from build123d import *

# Parameters (mm, degrees)
F1_DEPTH    = 2.5
F3_DEPTH    = 2.7
F4_R        = 1
F5_R        = 5
F7_R        = 2
F8_DEPTH    = 1
F6_W        = 8
F6_H        = 15
F9_DEPTH    = 1.1
F10_SIZE2   = 1.09999
F10_SIZE    = 14.99999
F10_2_SIZE2 = 1.09999
F10_2_SIZE  = 14.99999
F13_W       = 4
F13_H       = 4
F14_DEPTH   = 2


# Not quite as in the source:
# - a fillet or chamfer that OpenCascade refuses, or shapes differently, is made with other operations: its cross-section is extruded or revolved along the edge and cut away or added
# - two fillets or chamfers of one size are made in one step
# - a fillet or chamfer is up to 0.001 mm smaller than in the source, because OpenCascade refuses the exact size


with BuildPart() as f1:
    # F0 (on Top) → F1 (new body)
    with BuildSketch(Plane.XY):
        Polygon((55, 0), (4, 0), (0, -10), (0, -47), (59, -47), (59, -10), align=None)
    extrude(amount=F1_DEPTH)

    # F2 (on face) → F3 (join)
    with BuildSketch(Plane.XY.offset(2.5)):
        with BuildLine():
            Line((0, -39.5), (0, -47))
            Line((0, -47), (59, -47))
            Line((59, -47), (59, -39.5))
            Line((59, -39.5), (53.5, -32))
            Line((53.5, -32), (53.5, -4))
            ThreePointArc((53.5, -4), (52.3284271247, -1.1715728753), (49.5, 0))
            Line((49.5, 0), (9.5, 0))
            ThreePointArc((9.5, 0), (6.6715728753, -1.1715728753), (5.5, -4))
            Line((5.5, -4), (5.5, -32))
            Line((5.5, -32), (0, -39.5))
        make_face()
    extrude(amount=F3_DEPTH)

    # F4
    f4_edges = [f1.edges().sort_by_distance(p)[0] for p in [
        (0, -47, 2.6),
        (59, -47, 2.6),
        (4, 0, 1.25),
        (55, 0, 1.25),
        (59, -10, 1.25),
        (0, -10, 1.25),
    ]]
    fillet(f4_edges, radius=F4_R)

    # F5
    f5_edges = [f1.edges().sort_by_distance(p)[0] for p in [
        (0, -39.5, 3.85),
        (59, -39.5, 3.85),
        (53.5, -32, 3.85),
        (5.5, -32, 3.85),
    ]]
    fillet(f5_edges, radius=F5_R)

    # F7 (on face) → F8 (cut)
    with BuildSketch(Plane(origin=(0, 0, 0), x_dir=(1, 0, 0), z_dir=(0, 0, -1))):
        with Locations((19, 20)):
            Circle(F7_R)
        with Locations((40, 20)):
            Circle(F7_R)
    extrude(amount=-F8_DEPTH, mode=Mode.SUBTRACT)

    # F6 (on face) → F9 (cut)
    with BuildSketch(Plane(origin=(0, 0, 0), x_dir=(1, 0, 0), z_dir=(0, 0, -1))):
        with Locations((40, 7.5)):
            Rectangle(F6_W, F6_H)
        with Locations((19, 7.5)):
            Rectangle(F6_W, F6_H)
    extrude(amount=-F9_DEPTH, mode=Mode.SUBTRACT)

    # F10 (size 15 and 1.1 in the source; OpenCascade refuses exactly that, so slightly less here)
    f10_edges = [f1.edges().sort_by_distance(p)[0] for p in [
        (40, -15, 1.1),
    ]]
    f10_side = f1.faces().sort_by_distance((40, -7.5, 1.1))[0]
    chamfer(f10_edges, length=F10_SIZE, length2=F10_SIZE2, reference=f10_side)

    # F10#2 (size 15 and 1.1 in the source; OpenCascade refuses exactly that, so slightly less here)
    f10_2_edges = [f1.edges().sort_by_distance(p)[0] for p in [
        (19, -15, 1.1),
    ]]
    f10_2_side = f1.faces().sort_by_distance((19, -7.5, 1.1))[0]
    chamfer(f10_2_edges, length=F10_2_SIZE, length2=F10_2_SIZE2, reference=f10_2_side)

    # F12: fillet of radius 2 on 2 edges, made by hand

    # F12_s1 → F12_t2 (revolve)
    with BuildSketch(Plane.XZ.offset(20)):
        with BuildLine():
            ThreePointArc((42, 0), (41.2679491924, 0.7320508076), (40.2679491924, 1))
            Line((40.2679491924, 1), (42, 1))
            Line((42, 1), (42, 0))
        make_face()
    revolve(axis=Axis((40, -20, 1), (0, 0, -1)))

    # F12_s3 → F12_t4 (revolve)
    with BuildSketch(Plane.XZ.offset(20)):
        with BuildLine():
            ThreePointArc((21, 0), (20.2679491924, 0.7320508076), (19.2679491924, 1))
            Line((19.2679491924, 1), (21, 1))
            Line((21, 1), (21, 0))
        make_face()
    revolve(axis=Axis((19, -20, 1), (0, 0, -1)))

    # F13 (on face) → F14 (join)
    with BuildSketch(Plane.XY.offset(5.2)):
        with Locations((11.5, -6)):
            Rectangle(F13_W, F13_H)
        with Locations((11.5, -41)):
            Rectangle(F13_W, F13_H)
        with Locations((47.5, -6)):
            Rectangle(F13_W, F13_H)
        with Locations((47.5, -41)):
            Rectangle(F13_W, F13_H)
    extrude(amount=F14_DEPTH)


solid = f1.part
Could you check a few things on this model? Use its own coordinates, in mm. A direction names the side the tool comes from. Give positions to 0.01 mm unless a question says otherwise; leave off trailing zeros. Loops run counter-clockwise (first coordinate to the right, second up) from the corner with the lowest first, then second, coordinate; pieces in that order, holes last. Notation, with made-up numbers: M 78,-9.75 L 91,-9.75 A27 cw 91,27.25 Z; hole C 11,-34.5 d1. An arc over 180 degrees is marked long. Answer as a JSON object with one key per item and string values.
Q1. If we mould it in two halves opening along X, with no side actions, what happens to faces 1 (the flat face through (13.5, -41, 6)), 2 (the flat face through (9.5, -6, 6)), 3 (the flat face through (29, -23, 0))? For each: pulls with the +X half, pulls with the -X half, needs draft (parallel to the pull), parting line crosses it, or undercut.
Values found:
{"face 1": "undercut", "face 2": "pulls with the -X half", "face 3": "needs draft"}
Q2. For P1, Ø0.6, axis at x = 12.5, z = 6.5, coming from the -Y side; P2, Ø1.6, axis at y = -7, z = 6.5, coming from the -X side; P3, Ø1, axis at x = 47.5, z = 6.5, coming from the +Y side, each with a flat end and sliding along its axis, tell me the tip position at first contact or that it passes through.
Values found:
{"P1": "stops at y = -43", "P2": "stops at x = 9.5", "P3": "stops at y = -4"}
Q3. Suppose I cut it at C-C, the plane y = -28.5. List the corners of the cut face in (x, z) for me, plus the area to 3 significant figures.
Values found:
{"outline": "M 0,0 L 59,0 L 59,2.5 L 53.5,2.5 L 53.5,5.2 L 5.5,5.2 L 5.5,2.5 L 0,2.5 Z", "area": "277 mm²"}
Q4. If I drill on probe 1 along X at (y, z) = (-40.5, 6.75); probe 2 along Z at (x, y) = (30.5, -11); probe 3 along Y at (x, z) = (48, 6.5), over which ranges is the centre line in solid material (lowest first)? Write a range as [from, to].
Values found:
{"probe 1": "x = [9.5, 13.5], [45.5, 49.5]", "probe 2": "z = [0, 5.2]", "probe 3": "y = [-43, -39], [-8, -4]"}
Q5. Suppose I cut it at D-D, the plane y = -9. List the corners of the cut face in (x, z) for me.
Values found:
{"outline": "M 0.4,0 L 15,0 L 15,0.44 L 23,0.44 L 23,0 L 36,0 L 36,0.44 L 44,0.44 L 44,0 L 58.6,0 L 58.6,2.5 L 53.5,2.5 L 53.5,5.2 L 5.5,5.2 L 5.5,2.5 L 0.4,2.5 Z"}
Q6. Suppose I cut it at A-A, the plane z = 6.5. List the corners of the cut face in (x, y) for me, plus the area to 3 significant figures.
Values found:
{"outline": "M 9.5,-43 L 13.5,-43 L 13.5,-39 L 9.5,-39 Z; M 9.5,-8 L 13.5,-8 L 13.5,-4 L 9.5,-4 Z; M 45.5,-43 L 49.5,-43 L 49.5,-39 L 45.5,-39 Z; M 45.5,-8 L 49.5,-8 L 49.5,-4 L 45.5,-4 Z", "area": "64.0 mm²"}
Q7. For faces 4 (the flat face through (11, -43, 6)), 5 (the flat face through (18.94, -7.61, 0.54)), 6 (the cylindrical face through (52.359, -1.203, 3.831)), 7 (the cylindrical face through (5.245, -31.94, 3.869)), 8 (the flat face through (49.5, -6, 6)), which set-ups out of +Z, -Z, +X, -X, +Y, -Y let a thin tool reach every point of the face, with its end or its side?
Values found:
{"face 4": "+Z, +X, -X, -Y", "face 5": "-Z, +Y", "face 6": "+Z, +X, +Y", "face 7": "+Z, -X, +Y", "face 8": "+Z, +X, +Y, -Y"}
